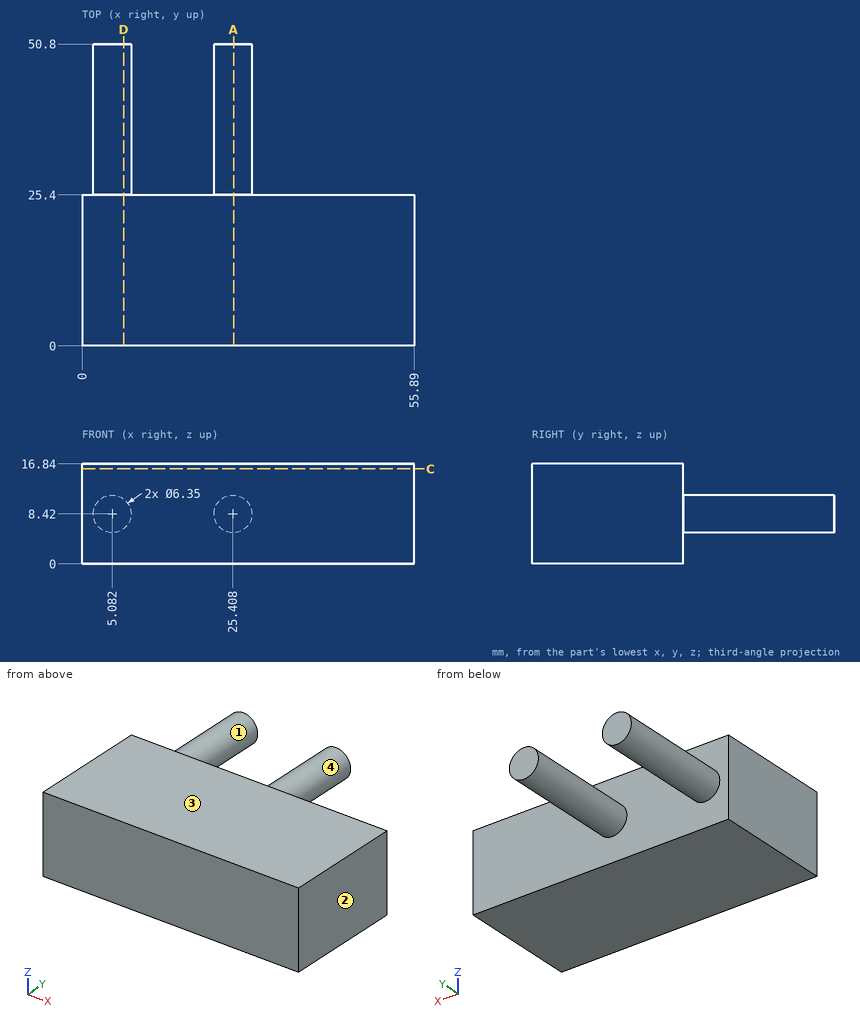
Geometry check sheet. Reference: drawing and pictorial views, mm from the part's lowest x, y, z. Coordinates: 2 decimals unless noted, no trailing zeros. Order: outer loops, then holes, each group sorted by start corner. A loop starts at its lowest first (then second) coordinate and runs counter-clockwise, first axis right, second up. Notation, with made-up numbers: (55, 46) - (84, 46) arc R35 ccw to (84, 79) - close; hole circle Ø10 at (43.5, 35). An arc over 180 degrees is marked (long way). Answer in a Markdown table with one row per item. Add a question column.
1) Material ranges on line 1 along Y through (x, z) = (46.5, 9.75); line 2 along X through (y, z) = (30, 5.5) (1 decimal); line 3 along X through (y, z) = (42.5, 9.5) (1 decimal), recorded low to high. Write a range as [from, to].
2) Cross-section at A-A, the plane x = 25.5. Record the cut outline in (y, z).
3) Release check for a two-part mould opening along X. For the marked faces 1, 2, 3 and 4 record: +X half, -X half, draft (parallel to the pull), parting line (faces both ways), or undercut.
4) Gauge pin test, flat ends, axial feed: P1, Ø12, axis at x = 33, y = 33.5, coming from the -Z side; P2, Ø4, axis at y = 32.5, z = 12.5, coming from the -X side; P3, Ø5, axis at x = 29.5, z = 13.5, coming from the +Y side. Record the tip position at first contact, or that the pin passes through.
5) Cross-section at D-D, the plane x = 7. Record the cut outline in (y, z).
6) Cross-section at C-C, the plane z = 16. Record the cut outline in (x, y).
Check result:
| question | item | result |
|---|---|---|
| 1 | line 1 | y = [0, 25.4] |
| 1 | line 2 | x = [3.8, 6.3], [24.2, 26.7] |
| 1 | line 3 | x = [2.1, 8.1], [22.4, 28.4] |
| 2 | outline | (0, 0) - (25.4, 0) - (25.4, 5.25) - (50.8, 5.25) - (50.8, 11.59) - (25.4, 11.59) - (25.4, 16.84) - (0, 16.84) - close |
| 3 | face 1 | undercut |
| 3 | face 2 | +X half |
| 3 | face 3 | draft |
| 3 | face 4 | undercut |
| 4 | P1 | stops at z = 5.67 |
| 4 | P2 | stops at x = 2.68 |
| 4 | P3 | stops at y = 25.4 |
| 5 | outline | (0, 0) - (25.4, 0) - (25.4, 5.89) - (50.8, 5.89) - (50.8, 10.95) - (25.4, 10.95) - (25.4, 16.84) - (0, 16.84) - close |
| 6 | outline | (0, 0) - (55.89, 0) - (55.89, 25.4) - (0, 25.4) - close |
